Design review of the part built by this model. Coordinates are the model's own, in mm. A direction names the side the tool comes from. Round coordinates to 2 decimals unless told otherwise and drop trailing zeros. Write each loop counter-clockwise with the first axis right and the second up, starting at its lowest first coordinate (ties: lowest second). Pieces come first, ordered by that corner, then holes. Notation, with made-up numbers: (37, 75) - (86, 75) arc R20 ccw to (86, 89) - close; hole circle Ø1 at (20, -7). An arc over 180 degrees is marked (long way). Use one line per item in the form item = value.
```python
from build123d import *

# Parameters (mm, degrees)
SKETCH_1_W      = 56
SKETCH_1_H      = 65
EXTRUDE_1_DEPTH = 10
FILLET_1_R      = 4
FILLET_2_R      = 0.5
SKETCH_2_R      = 7
EXTRUDE_2_DEPTH = 2


with BuildPart() as part:
    # 草图1 → 凸台-拉伸1 (new body)
    with BuildSketch(Plane(origin=(0, 0, 0), x_dir=(1, 0, 0), z_dir=(0, 1, 0))):
        Rectangle(SKETCH_1_W, SKETCH_1_H)
    extrude(amount=EXTRUDE_1_DEPTH)

    # 圆角1
    fillet_1_edges = [part.edges().sort_by_distance(p)[0] for p in [
        (-28, 10, 0),
        (28, 10, 0),
        (-28, 0, 0),
        (28, 0, 0),
    ]]
    fillet(fillet_1_edges, radius=FILLET_1_R)

    # 圆角2
    fillet_2_edges = [part.edges().sort_by_distance(p)[0] for p in [
        (-28, 5, 32.5),
        (-28, 5, -32.5),
        (0, 0, 32.5),
        (28, 5, 32.5),
        (0, 10, 32.5),
        (-26.828427125, 8.828427125, 32.5),
        (26.828427125, 8.828427125, 32.5),
        (26.828427125, 1.171572875, 32.5),
        (-26.828427125, 1.171572875, 32.5),
        (0, 0, -32.5),
        (0, 10, -32.5),
        (28, 5, -32.5),
        (-26.828427125, 8.828427125, -32.5),
        (26.828427125, 8.828427125, -32.5),
        (26.828427125, 1.171572875, -32.5),
        (-26.828427125, 1.171572875, -32.5),
    ]]
    fillet(fillet_2_edges, radius=FILLET_2_R)

    # 草图2 → 凸台-拉伸2 (add)
    with BuildSketch(Plane.XZ):
        with Locations(Location((0, 6.105786748, 0), (0, 0, 90))):
            Circle(SKETCH_2_R)
    extrude(amount=EXTRUDE_2_DEPTH)


solid = part.part
```
Q1. For P1, Ø10, axis at x = -7, z = 25.5, coming from the -Y side, flat-tipped, find the tip position at first contact; note if it passes through.
Calculated:
P1 = 0
Q2. To check wall thickness, follow line 1 along Y through (x, z) = (9, -13.5); line 2 along X through (y, z) = (3, 22.5); line 3 along Y through (x, z) = (-25, -25). State the ranges of each line that lie inside material, in increasing order. Write a range as from..to.
Calculated:
line_1 = 0..10
line_2 = -27.87..27.87
line_3 = 0.13..9.87
Q3. Machinability: for faces 1 (the cylindrical face through (-0.308, -0.986, -0.887)), 2 (the cylindrical face through (-26.859, 1.203, -0.448)), which of the approach directions +Z, -Z, +X, -X, +Y, -Y give a long, thin tool a straight path to every point of the face, cutting with its end or side? Answer none if there is none.
Calculated:
face_1 = -Y
face_2 = +Z, -Z, -X, -Y
Q4. We need section A-A on x = 0. Write out the cut boundary in (y, z).
Calculated:
outline = (-2, -0.89) - (0, -0.89) - (0, -32) arc R0.5 ccw to (0.5, -32.5) - (9.5, -32.5) arc R0.5 ccw to (10, -32) - (10, 32) arc R0.5 ccw to (9.5, 32.5) - (0.5, 32.5) arc R0.5 ccw to (0, 32) - (0, 13.11) - (-2, 13.11) - close
Q5. We need section B-B on z = -16.5. Write out the cut boundary in (x, y).
Calculated:
outline = (-28, 4) arc R4 ccw to (-24, 0) - (24, 0) arc R4 ccw to (28, 4) - (28, 6) arc R4 ccw to (24, 10) - (-24, 10) arc R4 ccw to (-28, 6) - close
